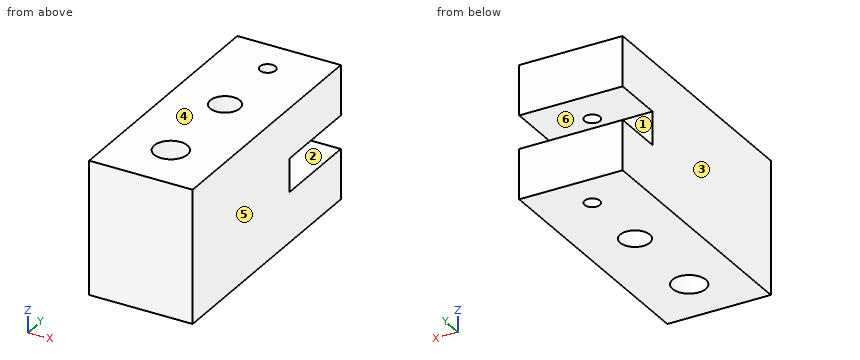
```python
from build123d import *

# Parameters (mm, degrees)
SKETCH2_W           = 14
SKETCH2_H           = 34.7
BOSS_EXTRUDE1_DEPTH = 18
SKETCH3_R           = 2.25
SKETCH3_R_2         = 2
CUT_EXTRUDE1_DEPTH  = 26.961943302
SKETCH4_W           = 4.5
SKETCH4_H           = 12
CUT_EXTRUDE2_DEPTH  = 8
SKETCH5_R           = 1.05
CUT_EXTRUDE3_DEPTH  = 26.961943302
SKETCH8_W           = 4.5
SKETCH8_H           = 7
CUT_EXTRUDE6_DEPTH  = 29.653490189


with BuildPart() as part:
    # Sketch2 → Boss-Extrude1 (new body)
    with BuildSketch(Plane.XY):
        Rectangle(SKETCH2_W, SKETCH2_H)
    extrude(amount=BOSS_EXTRUDE1_DEPTH)

    # Sketch3 → Cut-Extrude1 (cut, through all)
    with BuildSketch(Plane.XY.offset(18)):
        with Locations((0, -10.35)):
            Circle(SKETCH3_R)
        with Locations((0, 2.35)):
            Circle(SKETCH3_R_2)
    extrude(amount=-CUT_EXTRUDE1_DEPTH, mode=Mode.SUBTRACT)

    # Sketch4 → Cut-Extrude2 (cut)
    with BuildSketch(Plane(origin=(7, 0, 0), x_dir=(0, 0, -1), z_dir=(1, 0, 0))):
        with Locations((-9, 11.35)):
            Rectangle(SKETCH4_W, SKETCH4_H)
    extrude(amount=-CUT_EXTRUDE2_DEPTH, mode=Mode.SUBTRACT)

    # Sketch5 → Cut-Extrude3 (cut, through all)
    with BuildSketch(Plane.XY.offset(18)):
        with Locations((0, 12.35)):
            Circle(SKETCH5_R)
    extrude(amount=-CUT_EXTRUDE3_DEPTH, mode=Mode.SUBTRACT)

    # Sketch8 → Cut-Extrude6 (cut, through all)
    with BuildSketch(Plane(origin=(7, 0, 0), x_dir=(0, 0, -1), z_dir=(1, 0, 0))):
        with Locations((-9, 13.85)):
            Rectangle(SKETCH8_W, SKETCH8_H)
    extrude(amount=-CUT_EXTRUDE6_DEPTH, mode=Mode.SUBTRACT)


solid = part.part
```
For this review, take the finished solid that the model builds, in its own axes (mm). Face numbers are marked on the shaded views. A direction names the side the tool comes from. Give positions to 0.01 mm unless a question says otherwise; leave off trailing zeros. Loops run counter-clockwise (first coordinate to the right, second up) from the corner with the lowest first, then second, coordinate; pieces in that order, holes last. Notation, with made-up numbers: M 88.25,22.5 L 134.25,22.5 A24 ccw 134.25,40.5 Z; hole C -3,89 d4. An arc over 180 degrees is marked long. One line per item, written item: value. Start each with the question number.
Q1. Add section A-A (y = 2.35). Give the boundary of the cut face in (x, z), and give its area (3 significant figures).
Q2. Draft analysis for pull direction Z (two halves, no side actions). For the marked faces 4, 5 and 6, state which applies: released by +Z, released by -Z, zero draft, split by the parting line, or undercut.
Q3. Add section D-D (x = 0). Give the boundary of the cut face in (y, z), and give its area (3 significant figures).
Q4. Machinability: for the marked faces 1, 2 and 3, which of the approach directions +Z, -Z, +X, -X, +Y, -Y give a long, thin tool a straight path to every point of the face, cutting with its end or side? Answer none if there is none.
Q5. Add section C-C (y = 12.35). Give the boundary of the cut face in (x, z), and give its area (3 significant figures).
Q6. Clearance check with flat-ended pins moving along their axes: pin 1 Ø2 at (y, z) = (8.5, 8.5) entering from +X; pin 2 Ø2 at (x, z) = (-5, 9) entering from +Y; pin 3 Ø2 at (x, z) = (2, 9) entering from +Y. State where each tip first meets the part, or that it passes through.
Q7. Add section B-B (z = 9.75). Give the boundary of the cut face in (x, y), and give its area (3 significant figures).
Q8. For L1, parallel to Y at x = 0, z = 10.75; L2, parallel to Y at x = 0, z = 12; L3, parallel to Z at x = 1.75, y = 14, list the stretches that pass through material, from the lowest coordinate up.
Reply:
1. outline: M -7,0 L -2,0 L -2,18 L -7,18 Z; M 2,0 L 7,0 L 7,18 L 2,18 Z
1. area: 180 mm²
2. face 4: released by +Z
2. face 5: zero draft
2. face 6: undercut
3. outline: M -17.35,0 L -12.6,0 L -12.6,18 L -17.35,18 Z; M -8.1,0 L 0.35,0 L 0.35,18 L -8.1,18 Z; M 4.35,0 L 11.3,0 L 11.3,6.75 L 5.35,6.75 L 5.35,11.25 L 11.3,11.25 L 11.3,18 L 4.35,18 Z; M 13.4,0 L 17.35,0 L 17.35,6.75 L 13.4,6.75 Z; M 13.4,11.25 L 17.35,11.25 L 17.35,18 L 13.4,18 Z
3. area: 389 mm²
4. face 1: +X, -X, +Y
4. face 2: +X, +Y
4. face 3: +Z, -Z, -X, +Y, -Y
5. outline: M -7,0 L -1.05,0 L -1.05,6.75 L -7,6.75 Z; M -7,11.25 L -1.05,11.25 L -1.05,18 L -7,18 Z; M 1.05,0 L 7,0 L 7,6.75 L 1.05,6.75 Z; M 1.05,11.25 L 7,11.25 L 7,18 L 1.05,18 Z
5. area: 161 mm²
6. pin 1: x = -1
6. pin 2: y = 10.35
6. pin 3: y = 5.35
7. outline: M -7,-17.35 L 7,-17.35 L 7,5.35 L -1,5.35 L -1,10.35 L -7,10.35 Z; hole C 0,-10.35 d4.5; hole C 0,2.35 d4
7. area: 319 mm²
8. L1: -17.35 to -12.6, -8.1 to 0.35, 4.35 to 5.35
8. L2: -17.35 to -12.6, -8.1 to 0.35, 4.35 to 11.3, 13.4 to 17.35
8. L3: 0 to 6.75, 11.25 to 18
